For this review, take the finished solid that the model builds, in its own axes (mm). Face numbers are marked on the shaded views. A direction names the side the tool comes from. Round coordinates to 2 decimals unless told otherwise and drop trailing zeros. Write each loop counter-clockwise with the first axis right and the second up, starting at its lowest first coordinate (ties: lowest second). Pieces come first, ordered by that corner, then holes. Notation, with made-up numbers: (60, 27) - (94, 27) arc R22 cw to (94, 66) - close; hole circle Ø11 at (87, 6.25). An arc over 180 degrees is marked (long way). One line per item, written item: value. Start each with the question number.
Q1. Mouldability with a two-part tool opening along Z and no side actions: class the marked faces 1, 2 and 3 as +Z half, -Z half, draft (parallel to the pull), parting line (faces both ways), or undercut.
Q2. Add section D-D on y = -34. Write out the cut boundary in (x, z), and give its area (3 significant figures).
Q3. Add section B-B on x = 33.5. Write out the cut boundary in (y, z), and give its area (3 significant figures).
Q4. Add section C-C on z = 30.5. Write out the cut boundary in (x, y), and give its area (3 significant figures).
Q5. For probe 1 along Z at (x, y) = (39, -21); probe 2 along Z at (x, y) = (39, -48.5); probe 3 along Y at (x, z) = (37, 30), list the stretches that pass through material, from the lowest coordinate up.
Q6. Clearance check with flat-ended pins moving along their axes: pin 1 Ø5 at (x, z) = (39, 50) entering from +Y; pin 2 Ø3 at (x, z) = (40, 52) entering from -Y; pin 3 Ø1.5 at (x, y) = (43, -32) entering from +Z. State where each tip first meets the part, or that it passes through.
Q7. Tool access review of the marked faces 4, 5, 6, 7 and 8: name each direction out of +Z, -Z, +X, -X, +Y, -Y from which nothing blocks a thin tool from reaching the whole face with its end or side.
Q8. Add section A-A on y = 13.5. Write out the cut boundary in (x, z), and give its area (3 significant figures).
```python
from build123d import *

# Parameters (mm, degrees)
SKETCH1_R                                        = 0.9
SKETCH1_W                                        = 12
SKETCH1_H                                        = 23
BOSS_EXTRUDE1_DEPTH                              = 42
CBORE_FOR_M4_PAN_HEAD_MACHINE_SCREW2_D           = 4.5
CBORE_FOR_M4_PAN_HEAD_MACHINE_SCREW2_CBORE_D     = 9
CBORE_FOR_M4_PAN_HEAD_MACHINE_SCREW2_CBORE_DEPTH = 3.1
CUT_EXTRUDE2_DEPTH                               = 4
SKETCH11_W                                       = 35
SKETCH11_H                                       = 57
CUT_EXTRUDE3_DEPTH                               = 36
SKETCH12_W                                       = 24
SKETCH12_H                                       = 54
CUT_EXTRUDE4_DEPTH                               = 34
BOSS_EXTRUDE2_DEPTH                              = 8
BOSS_EXTRUDE2_DEPTH_BACK                         = 14
FILLET3_R                                        = 4
SKETCH14_W                                       = 8.2
SKETCH14_H                                       = 15
CUT_EXTRUDE5_DEPTH                               = 92.094527719
FILLET4_R                                        = 6
FILLET5_R                                        = 4
CUT_EXTRUDE6_DEPTH                               = 94.87574371
FILLET6_R                                        = 10


with BuildPart() as part:
    # Sketch1 → Boss-Extrude1 (new body)
    with BuildSketch(Plane(origin=(0, 0, 0), x_dir=(0, 0, -1), z_dir=(1, 0, 0))):
        with BuildLine():
            Line((-55.350295908, -42.411439664), (-43.208412731, -42.411439664))
            ThreePointArc((-43.208412731, -42.411439664), (-27.350295908, -43.911439664), (-43.208412731, -45.411439664))
            Line((-43.208412731, -45.411439664), (-55.350295908, -45.411439664))
            Line((-55.350295908, -45.411439664), (-55.350295908, -58.911439664))
            Line((-55.350295908, -58.911439664), (-20.350295908, -58.911439664))
            Line((-20.350295908, -58.911439664), (-20.350295908, -16.911439664))
            Line((-20.350295908, -16.911439664), (28.649704092, -16.911439664))
            Line((28.649704092, -16.911439664), (28.649704092, 37.088560336))
            Line((28.649704092, 37.088560336), (4.649704092, 37.088560336))
            Line((4.649704092, 37.088560336), (4.649704092, -1.911439664))
            Line((4.649704092, -1.911439664), (-55.350295908, -1.911439664))
            Line((-55.350295908, -1.911439664), (-55.350295908, -28.911439664))
            Line((-55.350295908, -28.911439664), (-55.350295908, -42.411439664))
        make_face()
        with Locations(Location((16.649704092, 34.088560336, 0), (0, 0, 180))):
            Circle(SKETCH1_R, mode=Mode.SUBTRACT)
        with Locations(Location((16.649704092, 5.088560336, 0), (0, 0, 180))):
            Circle(SKETCH1_R, mode=Mode.SUBTRACT)
        with Locations((16.649704092, 19.588560336)):
            Rectangle(SKETCH1_W, SKETCH1_H, mode=Mode.SUBTRACT)
    extrude(amount=BOSS_EXTRUDE1_DEPTH)

    # CBORE for M4 Pan Head Machine Screw2 (through all)
    with Locations(Plane(origin=(0, -58.911439664, 0), x_dir=(-1, 0, 0), z_dir=(0, -1, 0))):
        with Locations((-39, -49.450295908)):
            CounterBoreHole(CBORE_FOR_M4_PAN_HEAD_MACHINE_SCREW2_D / 2, CBORE_FOR_M4_PAN_HEAD_MACHINE_SCREW2_CBORE_D / 2, CBORE_FOR_M4_PAN_HEAD_MACHINE_SCREW2_CBORE_DEPTH)

    # Sketch7 → Cut-Extrude2 (cut)
    with BuildSketch(Plane(origin=(0, -1.911439664, 0), x_dir=(1, 0, 0), z_dir=(0, 1, 0))):
        Polygon((42.55, -51.499889363), (42.55, -47.400702452), (39, -45.351108997), (35.45, -47.400702452), (35.45, -51.499889363), (39, -53.549482819), align=None)
    extrude(amount=-CUT_EXTRUDE2_DEPTH, mode=Mode.SUBTRACT)

    # Sketch11 → Cut-Extrude3 (cut)
    with BuildSketch(Plane.ZY):
        with Locations((37.850295908, -30.411439664)):
            Rectangle(SKETCH11_W, SKETCH11_H)
    extrude(amount=-CUT_EXTRUDE3_DEPTH, mode=Mode.SUBTRACT)

    # Sketch12 → Cut-Extrude4 (cut)
    with BuildSketch(Plane(origin=(42, 0, 0), x_dir=(0, 0, -1), z_dir=(1, 0, 0))):
        with Locations((16.649704092, 10.088560336)):
            Rectangle(SKETCH12_W, SKETCH12_H)
    extrude(amount=-CUT_EXTRUDE4_DEPTH, mode=Mode.SUBTRACT)

    # Sketch13 → Boss-Extrude2 (add, two sides: drawn at the far end of the back side and taken through both)
    with BuildSketch(Plane.ZY.offset(-36).offset(-BOSS_EXTRUDE2_DEPTH_BACK)):
        with BuildLine():
            Line((40.350295908, -37.666441665), (40.350295908, -26.440452892))
            Line((40.350295908, -26.440452892), (20.350295908, -26.440452892))
            Line((20.350295908, -26.440452892), (20.350295908, -58.911439664))
            Line((20.350295908, -58.911439664), (41.134513551, -58.911439664))
            Line((41.134513551, -58.911439664), (41.134513551, -49.437996119))
            ThreePointArc((41.134513551, -49.437996119), (27.36798978, -44.443218651), (40.350295908, -37.666441665))
        make_face()
    extrude(amount=BOSS_EXTRUDE2_DEPTH + BOSS_EXTRUDE2_DEPTH_BACK)

    # Fillet3
    fillet3_edges = [part.edges().sort_by_distance(p)[0] for p in [
        (32, -58.911439664, 41.134513551),
        (32, -26.440452892, 20.350295908),
        (32, -26.440452892, 40.350295908),
        (46, -58.911439664, 41.134513551),
        (50, -42.675946278, 20.350295908),
        (46, -26.440452892, 20.350295908),
        (46, -26.440452892, 40.350295908),
        (28, -42.675946278, 20.350295908),
        (39, -58.911439664, 20.350295908),
    ]]
    fillet(fillet3_edges, radius=FILLET3_R)

    # Sketch14 → Cut-Extrude5 (cut, through all)
    with BuildSketch(Plane(origin=(42, 0, 0), x_dir=(0, 0, -1), z_dir=(1, 0, 0))):
        with Locations((-51.250295908, -34.911439664)):
            Rectangle(SKETCH14_W, SKETCH14_H)
    extrude(amount=-CUT_EXTRUDE5_DEPTH, mode=Mode.SUBTRACT)

    # Fillet4
    fillet4_edges = [part.edges().sort_by_distance(p)[0] for p in [
        (4, 37.088560336, -4.649704092),
        (4, 37.088560336, -28.649704092),
    ]]
    fillet(fillet4_edges, radius=FILLET4_R)

    # Fillet5
    # the kernel refuses this fillet: 4 mm, written as the material it takes off along each edge
    with BuildSketch(Plane(origin=(0, 31.088560336, -4.649704092), x_dir=(0, 0, -1), z_dir=(0, -1, 0))) as fillet5_piece_1:
        with BuildLine():
            CenterArc((FILLET5_R, FILLET5_R), FILLET5_R, 180, 90)
            Line((0, FILLET5_R), (0, 0))
            Line((0, 0), (FILLET5_R, 0))
        make_face()
    extrude(amount=33, mode=Mode.SUBTRACT)
    with BuildSketch(Plane(origin=(0, 31.088560336, -10.649704092), x_dir=(0, 0, 1), z_dir=(0, -1, 0))) as fillet5_piece_2:
        with BuildLine():
            CenterArc((6 - FILLET5_R, -FILLET5_R), FILLET5_R, 0, 90)
            Line((6, -FILLET5_R), (6, 0))
            Line((6, 0), (6 - FILLET5_R, 0))
        make_face()
    revolve(axis=Axis((0, 31.088560336, -10.649704092), (-1, 0, 0)), revolution_arc=90, mode=Mode.SUBTRACT)
    with BuildSketch(Plane(origin=(0, 37.088560336, -22.649704092), x_dir=(0, -1, 0), z_dir=(0, 0, 1))) as fillet5_piece_3:
        with BuildLine():
            CenterArc((FILLET5_R, FILLET5_R), FILLET5_R, 180, 90)
            Line((0, FILLET5_R), (0, 0))
            Line((0, 0), (FILLET5_R, 0))
        make_face()
    extrude(amount=12, mode=Mode.SUBTRACT)
    with BuildSketch(Plane(origin=(0, 31.088560336, -22.649704092), x_dir=(0, 0, -1), z_dir=(0, -1, 0))) as fillet5_piece_4:
        with BuildLine():
            CenterArc((6 - FILLET5_R, FILLET5_R), FILLET5_R, 270, 90)
            Line((6, FILLET5_R), (6, 0))
            Line((6, 0), (6 - FILLET5_R, 0))
        make_face()
    revolve(axis=Axis((0, 31.088560336, -22.649704092), (1, 0, 0)), revolution_arc=90, mode=Mode.SUBTRACT)
    with BuildSketch(Plane(origin=(8, -1.911439664, -4.649704092), x_dir=(-1, 0, 0), z_dir=(0, 1, 0))) as fillet5_piece_5:
        with BuildLine():
            CenterArc((FILLET5_R, -FILLET5_R), FILLET5_R, 90, 90)
            Line((0, -FILLET5_R), (0, 0))
            Line((0, 0), (FILLET5_R, 0))
        make_face()
    extrude(amount=33, mode=Mode.SUBTRACT)
    with BuildSketch(Plane(origin=(8, 31.088560336, -10.649704092), x_dir=(0, 0, 1), z_dir=(0, -1, 0))) as fillet5_piece_6:
        with BuildLine():
            CenterArc((6 - FILLET5_R, FILLET5_R), FILLET5_R, 270, 90)
            Line((6 - FILLET5_R, 0), (6, 0))
            Line((6, 0), (6, FILLET5_R))
        make_face()
    revolve(axis=Axis((8, 31.088560336, -10.649704092), (-1, 0, 0)), revolution_arc=90, mode=Mode.SUBTRACT)
    with BuildSketch(Plane(origin=(8, 37.088560336, -10.649704092), x_dir=(-1, 0, 0), z_dir=(0, 0, -1))) as fillet5_piece_7:
        with BuildLine():
            CenterArc((FILLET5_R, -FILLET5_R), FILLET5_R, 90, 90)
            Line((0, -FILLET5_R), (0, 0))
            Line((0, 0), (FILLET5_R, 0))
        make_face()
    extrude(amount=12, mode=Mode.SUBTRACT)
    with BuildSketch(Plane(origin=(8, 31.088560336, -22.649704092), x_dir=(0, 0, -1), z_dir=(0, -1, 0))) as fillet5_piece_8:
        with BuildLine():
            CenterArc((6 - FILLET5_R, -FILLET5_R), FILLET5_R, 0, 90)
            Line((6 - FILLET5_R, 0), (6, 0))
            Line((6, 0), (6, -FILLET5_R))
        make_face()
    revolve(axis=Axis((8, 31.088560336, -22.649704092), (1, 0, 0)), revolution_arc=90, mode=Mode.SUBTRACT)
    with BuildSketch(Plane(origin=(0, -26.911439664, -28.649704092), x_dir=(0, 0, 1), z_dir=(0, 1, 0))) as fillet5_piece_9:
        with BuildLine():
            CenterArc((FILLET5_R, FILLET5_R), FILLET5_R, 180, 90)
            Line((0, FILLET5_R), (0, 0))
            Line((0, 0), (FILLET5_R, 0))
        make_face()
    extrude(amount=58, mode=Mode.SUBTRACT)
    with BuildSketch(Plane(origin=(8, 31.088560336, -28.649704092), x_dir=(-1, 0, 0), z_dir=(0, -1, 0))) as fillet5_piece_10:
        with BuildLine():
            CenterArc((FILLET5_R, -FILLET5_R), FILLET5_R, 90, 90)
            Line((0, -FILLET5_R), (0, 0))
            Line((0, 0), (FILLET5_R, 0))
        make_face()
    extrude(amount=58, mode=Mode.SUBTRACT)
    with BuildSketch(Plane(origin=(-10, -16.911439664, -28.649704092), x_dir=(0, 1, 0), z_dir=(1, 0, 0))) as fillet5_piece_11:
        with BuildLine():
            CenterArc((FILLET5_R, FILLET5_R), FILLET5_R, 180, 90)
            Line((0, FILLET5_R), (0, 0))
            Line((0, 0), (FILLET5_R, 0))
        make_face()
    extrude(amount=28, mode=Mode.SUBTRACT)

    # Sketch15 → Cut-Extrude6 (cut, through all)
    with BuildSketch(Plane(origin=(0, -1.911439664, 0), x_dir=(1, 0, 0), z_dir=(0, 1, 0))):
        Polygon((36, -20.350295908), (0, -1.350295908), (0, -20.350295908), align=None)
        Polygon((8, 4.649704092), (42, -14.350295908), (42, 4.649704092), align=None)
    extrude(amount=-CUT_EXTRUDE6_DEPTH, mode=Mode.SUBTRACT)

    # Fillet6
    fillet6_edges = [part.edges().sort_by_distance(p)[0] for p in [
        (36, -9.411439664, 20.350295908),
        (0, -9.411439664, 1.350295908),
        (42, -9.411439664, 14.350295908),
    ]]
    fillet(fillet6_edges, radius=FILLET6_R)


solid = part.part
```
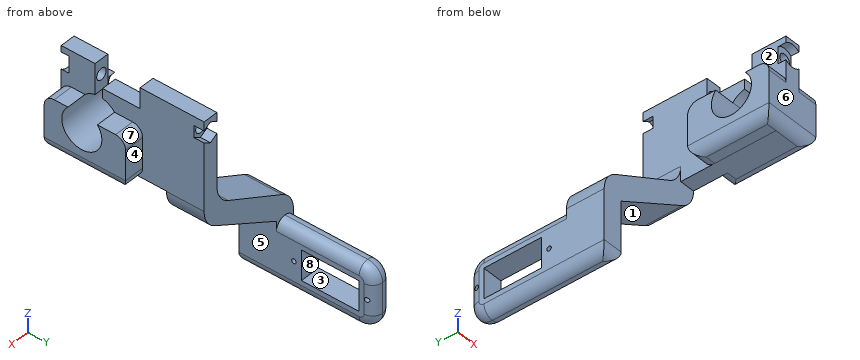
Result set:
1. face 1: -Z half
1. face 2: draft
1. face 3: undercut
2. outline: (28, 24.35) arc R4 ccw to (32, 20.35) - (46, 20.35) arc R4 ccw to (50, 24.35) - (50, 40.35) - (42, 40.35) - (42, 47.15) - (36, 47.15) - (36, 40.35) - (28, 40.35) - close
2. area: 474 mm^2
3. outline: (-58.91, 24.35) arc R4 ccw to (-54.91, 20.35) - (-30.44, 20.35) arc R4 ccw to (-26.44, 24.35) - (-26.44, 36.35) arc R4 ccw to (-30.44, 40.35) - (-37.67, 40.35) arc R8 cw (long way) to (-49.44, 41.13) - (-54.91, 41.13) arc R4 ccw to (-58.91, 37.13) - close; (-16.91, 9.6) - (-1.91, 9.6) - (-1.91, 19.77) - (-16.91, 19.77) - close
3. area: 620 mm^2
4. outline: (28, -58.91) - (50, -58.91) - (50, -50.27) - (28, -50.27) - close; (28, -37.55) - (50, -37.55) - (50, -26.44) - (42, -26.44) - (42, -1.91) - (36, -1.91) - (36, -26.44) - (28, -26.44) - close
4. area: 582 mm^2
5. probe 1: z = 20.35 to 47.2, 51.7 to 55.35
5. probe 2: z = 20.35 to 28.8, 41.9 to 47.2, 51.7 to 55.35
5. probe 3: y = -58.91 to -49.86, -37.96 to -1.91
6. pin 1: stops at y = -5.91
6. pin 2: stops at y = -55.81
6. pin 3: stops at z = 40.35
7. face 4: +Z, -Z, +X, +Y
7. face 5: -Z, +X, +Y, -Y
7. face 6: +Z, -Z, +X, -X, -Y
7. face 7: +Z, +X, +Y
7. face 8: +X, -X
8. outline: (0, -24.65) arc R4 ccw to (8, -24.65) - (8, -22.65) - (0, -22.65) - close; (0, -10.65) - (8, -10.65) - (8, -8.65) arc R4 ccw to (0, -8.65) - close
8. area: 82.3 mm^2
